The listing builds one solid part. Answer for the finished solid, in the listing's coordinates (mm). Face numbers are marked on the shaded views. A direction names the side the tool comes from. Round coordinates to 2 decimals unless told otherwise and drop trailing zeros. Loops run counter-clockwise (first coordinate to the right, second up) from the corner with the lowest first, then second, coordinate; pieces in that order, holes last. Notation, with made-up numbers: (44.25, 62) -> (97.25, 62) arc R17 cw to (97.25, 75) -> close; hole circle Ø2 at (68, 63). An arc over 180 degrees is marked (long way). Write each question's results on one line, items separated by ' | '. Start each with the question number.
(1) For the marked faces 1 and 2, determine the directions among +Z, -Z, +X, -X, +Y, -Y from which every point of the face is accessible in a straight line to the end or side of a thin tool.
(2) Flat-ended cylindrical pins translate along their axes: pin 1 (2 mm diameter, centred on x = 12, y = -7, fed in from +Z); pin 2 (2 mm diameter, centred on y = 4.5, z = -1.5, fed in from +X) (3 decimals); pin 3 (1.5 mm diameter, centred on y = -6, z = -1, fed in from -X); pin 4 (3 mm diameter, centred on x = -22.5, y = -13, fed in from +Z). Find the tip coordinate at first contact, or state that the pin passes through.
(3) Determine the mould class of the marked faces 3 and 4 for opening direction X: released by +X, released by -X, zero draft, split by the parting line, or undercut.
(4) Straight lines are drawn through the part: probe 1 along Z at (x, y) = (3.5, 12.5); probe 2 along Y at (x, z) = (-13.5, -2.25); probe 3 along Y at (x, z) = (13, 1.5). For each, find the intervals that lie inside material, in ascending order.
(5) The part is cut by section B-B (z = -1.75). Determine the outline of the cut face in (x, y).
(6) The part is cut by section A-A (z = 1.75). Determine the outline of the cut face in (x, y).
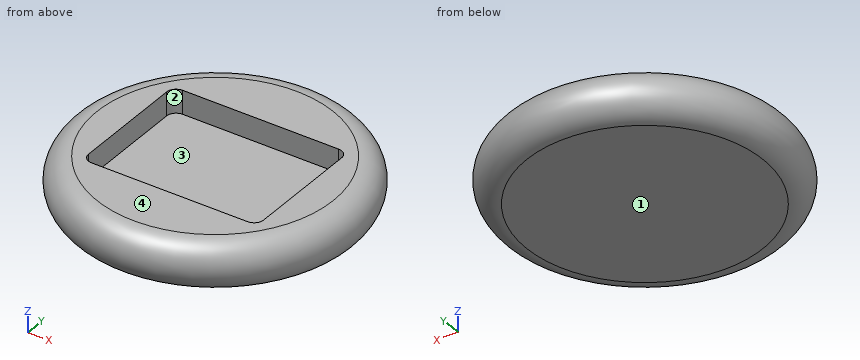
```python
from build123d import *

# Parameters (mm, degrees)
CUT_EXTRUDE3_DEPTH = 5


with BuildPart() as part:
    # Sketch7 → Revolve2 (revolve)
    with BuildSketch(Plane(origin=(0, 0, 0), x_dir=(1, 0, 0), z_dir=(0, 1, 0))):
        with BuildLine():
            Line((0, -2.5), (0, 7.5))
            Line((0, 7.5), (25, 7.5))
            ThreePointArc((25, 7.5), (30, 2.5), (25, -2.5))
            Line((25, -2.5), (0, -2.5))
        make_face()
    revolve(axis=Axis((0, 0, 2.5), (0, 0, -1)))

    # Sketch9 → Cut-Extrude3 (cut)
    with BuildSketch(Plane.XY.offset(2.5)):
        with BuildLine():
            Line((16.5, -14), (-16.5, -14))
            ThreePointArc((-16.5, -14), (-17.914213562, -13.414213562), (-18.5, -12))
            Line((-18.5, -12), (-18.5, 12))
            ThreePointArc((-18.5, 12), (-17.914213562, 13.414213562), (-16.5, 14))
            Line((-16.5, 14), (16.5, 14))
            ThreePointArc((16.5, 14), (17.914213562, 13.414213562), (18.5, 12))
            Line((18.5, 12), (18.5, -12))
            ThreePointArc((18.5, -12), (17.914213562, -13.414213562), (16.5, -14))
        make_face()
    extrude(amount=-CUT_EXTRUDE3_DEPTH, mode=Mode.SUBTRACT)


solid = part.part
```
Checked values:
1) face 1: -Z, +X, -X, +Y, -Y | face 2: +Z
2) pin 1: stops at z = -2.5 | pin 2: stops at x = 29.755 | pin 3: stops at x = -29.4 | pin 4: stops at z = 2.5
3) face 3: undercut | face 4: zero draft
4) probe 1: z = -7.5 to -2.5 | probe 2: y = -26.78 to -14, 14 to 26.78 | probe 3: y = -24.8 to -14, 14 to 24.8
5) outline: circle Ø59.89 at (0, 0); hole (-18.5, -12) arc R2 ccw to (-16.5, -14) -> (16.5, -14) arc R2 ccw to (18.5, -12) -> (18.5, 12) arc R2 ccw to (16.5, 14) -> (-16.5, 14) arc R2 ccw to (-18.5, 12) -> close
6) outline: circle Ø55.27 at (0, 0); hole (-18.5, -12) arc R2 ccw to (-16.5, -14) -> (16.5, -14) arc R2 ccw to (18.5, -12) -> (18.5, 12) arc R2 ccw to (16.5, 14) -> (-16.5, 14) arc R2 ccw to (-18.5, 12) -> close
